```python
from build123d import *

# Parameters (mm, degrees)
SKETCH_1_W           = 20
SKETCH_1_H           = 20
SKETCH_1_W_2         = 16
SKETCH_1_H_2         = 16
EXTRUDE_1_DEPTH      = 970
SKETCH_2_R           = 1
SKETCH_2_R_2         = 4.25
CUT_EXTRUDE_1_DEPTH  = 10
CUT_EXTRUDE_2_DEPTH  = 10
SKETCH_5_R           = 2.2
CUT_EXTRUDE_7_DEPTH  = 30
SKETCH_6_W           = 27.825743136
SKETCH_6_H           = 21.841712354
CUT_EXTRUDE_8_DEPTH  = 50
M4X0_7_3_D           = 3.3
M4X0_7_3_DEPTH       = 11.5
M4X0_7_3_TIP         = 0.991420021
SKETCH_11_R          = 1
CUT_EXTRUDE_9_DEPTH  = 10
M4X0_7_4_D           = 3.3
M4X0_7_4_DEPTH       = 11.5
M4X0_7_4_TIP         = 0.991420021
SKETCH_13_R          = 4.25
CUT_EXTRUDE_10_DEPTH = 21
M4X0_7_5_D           = 3.3
M4X0_7_5_DEPTH       = 11.5
M4X0_7_5_TIP         = 0.991420021


with BuildPart() as part:
    # ｽｹｯﾁ1 → ﾎﾞｽ - 押し出し1 (new body)
    with BuildSketch(Plane.XY):
        Rectangle(SKETCH_1_W, SKETCH_1_H)
        Rectangle(SKETCH_1_W_2, SKETCH_1_H_2, mode=Mode.SUBTRACT)
    extrude(amount=EXTRUDE_1_DEPTH)

    # ｽｹｯﾁ2 → ｶｯﾄ - 押し出し1 (cut)
    with BuildSketch(Plane(origin=(10, 0, 0), x_dir=(0, 0, -1), z_dir=(1, 0, 0))):
        with Locations((-710, 0)):
            Circle(SKETCH_2_R)
        with Locations((-50, 0)):
            Circle(SKETCH_2_R_2)
        with Locations((-40, 0)):
            Circle(SKETCH_2_R)
        with Locations((-730, 0)):
            Circle(SKETCH_2_R)
    extrude(amount=-CUT_EXTRUDE_1_DEPTH, mode=Mode.SUBTRACT)

    # ｽｹｯﾁ3 → ｶｯﾄ - 押し出し2 (cut)
    with BuildSketch(Plane(origin=(0, 10, 0), x_dir=(1, 0, 0), z_dir=(0, 1, 0))):
        with BuildLine():
            ThreePointArc((0, -649), (-1, -650), (0, -651))
            Line((0, -651), (0, -650))
            Line((0, -650), (0, -649))
        make_face()
        with BuildLine():
            Line((0, -650), (0, -651))
            ThreePointArc((0, -651), (0.707106781, -650.707106781), (1, -650))
            ThreePointArc((1, -650), (0.707106781, -649.292893219), (0, -649))
            Line((0, -649), (0, -650))
        make_face()
        with BuildLine():
            ThreePointArc((0, -669), (-1, -670), (0, -671))
            Line((0, -671), (0, -670))
            Line((0, -670), (0, -669))
        make_face()
        with BuildLine():
            Line((0, -670), (0, -671))
            ThreePointArc((0, -671), (0.707106781, -670.707106781), (1, -670))
            ThreePointArc((1, -670), (0.707106781, -669.292893219), (0, -669))
            Line((0, -669), (0, -670))
        make_face()
    extrude(amount=-CUT_EXTRUDE_2_DEPTH, mode=Mode.SUBTRACT)

    # ｽｹｯﾁ5 → ｶｯﾄ - 押し出し7 (cut)
    with BuildSketch(Plane(origin=(0, 10, 0), x_dir=(1, 0, 0), z_dir=(0, 1, 0))):
        with Locations((0, -117)):
            Circle(SKETCH_5_R)
        with Locations((0, -138)):
            Circle(SKETCH_5_R)
    extrude(amount=-CUT_EXTRUDE_7_DEPTH, mode=Mode.SUBTRACT)

    # ｽｹｯﾁ6 → ｶｯﾄ - 押し出し8 (cut)
    with BuildSketch(Plane.XY.offset(970)):
        Rectangle(SKETCH_6_W, SKETCH_6_H)
    extrude(amount=-CUT_EXTRUDE_8_DEPTH, mode=Mode.SUBTRACT)

    # M4x0.7 ねじ穴3
    with Locations(Plane(origin=(0, 10, 650), x_dir=(1, 0, 0), z_dir=(0, 1, 0))):
        with Locations((0, 0), (0, -20)):
            Hole(M4X0_7_3_D / 2, depth=M4X0_7_3_DEPTH)
            with Locations((0, 0, -(M4X0_7_3_DEPTH + M4X0_7_3_TIP / 2))):  # 118° drill point
                Cone(0, M4X0_7_3_D / 2, M4X0_7_3_TIP, mode=Mode.SUBTRACT)

    # ｽｹｯﾁ11 → ｶｯﾄ - 押し出し9 (cut)
    with BuildSketch(Plane(origin=(0, 10, 0), x_dir=(1, 0, 0), z_dir=(0, 1, 0))):
        with Locations((0, -30)):
            Circle(SKETCH_11_R)
        with Locations((0, -50)):
            Circle(SKETCH_11_R)
    extrude(amount=-CUT_EXTRUDE_9_DEPTH, mode=Mode.SUBTRACT)

    # M4x0.7 ねじ穴4
    with Locations(Plane(origin=(0, 10, 30), x_dir=(1, 0, 0), z_dir=(0, 1, 0))):
        with Locations((0, 0), (0, -20)):
            Hole(M4X0_7_4_D / 2, depth=M4X0_7_4_DEPTH)
            with Locations((0, 0, -(M4X0_7_4_DEPTH + M4X0_7_4_TIP / 2))):  # 118° drill point
                Cone(0, M4X0_7_4_D / 2, M4X0_7_4_TIP, mode=Mode.SUBTRACT)

    # ｽｹｯﾁ13 → ｶｯﾄ - 押し出し10 (cut, through all)
    with BuildSketch(Plane(origin=(10, 0, 0), x_dir=(0, 0, -1), z_dir=(1, 0, 0))):
        with Locations((-50, 0)):
            Circle(SKETCH_13_R)
    extrude(amount=-CUT_EXTRUDE_10_DEPTH, mode=Mode.SUBTRACT)

    # M4x0.7 ねじ穴5
    with Locations(Plane(origin=(10, 0, 40), x_dir=(0, 0, 1), z_dir=(1, 0, 0))):
        with Locations((0, 0), (670, 0), (690, 0)):
            Hole(M4X0_7_5_D / 2, depth=M4X0_7_5_DEPTH)
            with Locations((0, 0, -(M4X0_7_5_DEPTH + M4X0_7_5_TIP / 2))):  # 118° drill point
                Cone(0, M4X0_7_5_D / 2, M4X0_7_5_TIP, mode=Mode.SUBTRACT)


solid = part.part
```
Source: CAD feature listing. Evaluate the final solid. Frame: model axes, mm. A direction names the side the tool comes from. Round coordinates to 2 decimals unless told otherwise and drop trailing zeros. Order: outer loops, then holes, each group sorted by start corner. A loop starts at its lowest first (then second) coordinate and runs counter-clockwise, first axis right, second up. Notation, with made-up numbers: (-13, 59) -> (6, 59) arc R23 cw to (6, 83) -> close; hole circle Ø3 at (-7, 0). An arc over 180 degrees is marked (long way). One line per item, written item: value. Start each with the question number.
Q1. Access query for faces 4 (the flat face through (10, 0, 454)), 5 (the flat face through (8, 0, 454)). Directions: +Z, -Z, +X, -X, +Y, -Y. A direction counts if a zero-diameter tool reaches every point of the face in a straight line with its end or side. Return the directions, or none.
Q2. Section query A-A (z = 439). Return the cut outline in (x, y).
Q3. Pin query (flat end, axial travel): pin 1 (10 mm diameter, centred on x = -1.5, y = 7, fed in from +Z); pin 2 (2.5 mm diameter, centred on x = 0, z = 650, fed in from +Y). Return the tip coordinate at first contact, or that it passes through.
Q4. Material intervals for probe 1 along X at (y, z) = (8.55, 50); probe 2 along Y at (x, z) = (7.25, 491), sorted ascending.
Q5. Draft query along X for faces 1 (the flat face through (-10, 0, 454)), 2 (the flat face through (-9, 0, 0)), 3 (the flat face through (-8, 0, 454)). Return one class per face: pulls with the +X half, pulls with the -X half, needs draft (parallel to the pull), parting line crosses it, or undercut.
Findings below:
1. face 4: +Z, -Z, +X, +Y, -Y
1. face 5: +Z, -Z
2. outline: (-10, -10) -> (10, -10) -> (10, 10) -> (-10, 10) -> close; hole (-8, -8) -> (8, -8) -> (8, 8) -> (-8, 8) -> close
3. pin 1: z = 920
3. pin 2: y = -8
4. probe 1: -10 to -1.65, 1.65 to 10
4. probe 2: -10 to -8, 8 to 10
5. face 1: pulls with the -X half
5. face 2: needs draft
5. face 3: undercut
